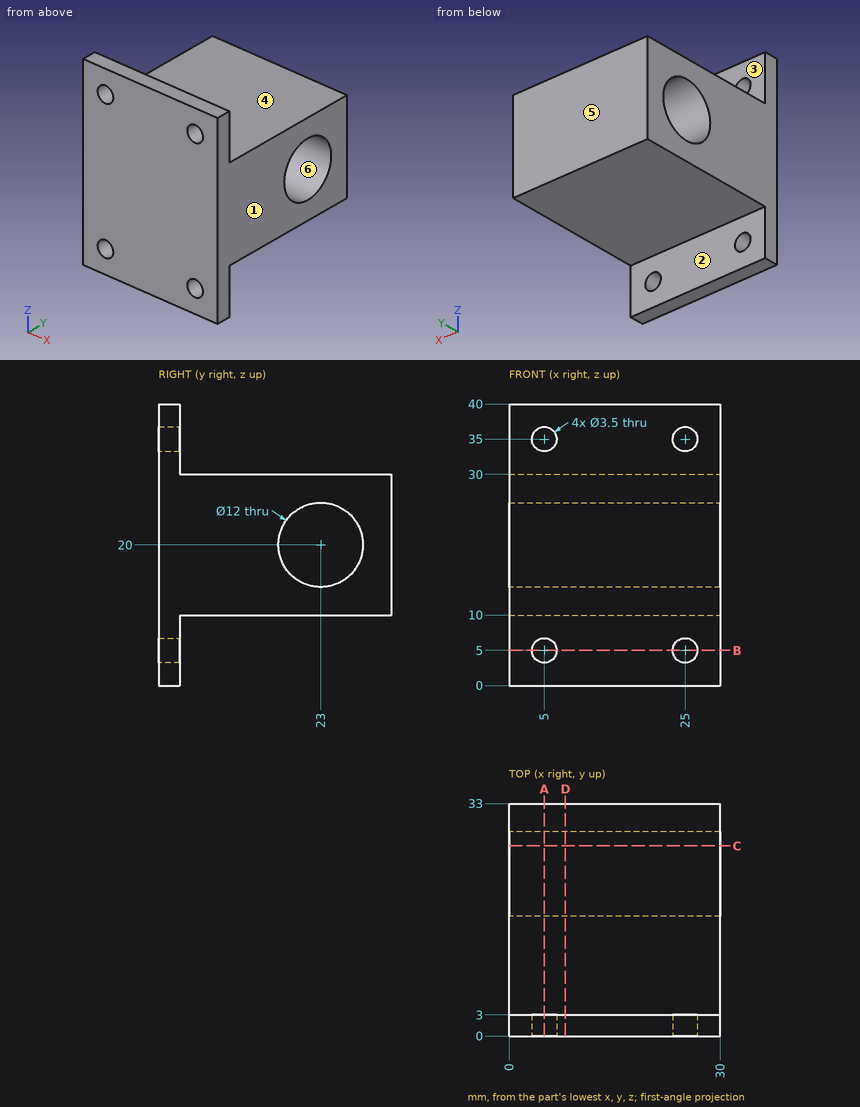
Check sheet for the drawn part. Datum: minimum x, y, z corner. Units: mm. A direction names the side the tool comes from. Coordinates: 2 decimals unless noted, no trailing zeros. Write each loop counter-clockwise with the first axis right and the second up, starting at its lowest first coordinate (ties: lowest second). Pieces come first, ordered by that corner, then holes. Notation, with made-up numbers: (-10, 85) - (46, 85) arc R21 ccw to (46, 100) - close; hole circle Ø7 at (26.25, 47.5). An arc over 180 degrees is marked (long way). Answer as a JSON object with one key per item and string values.
(1) Gauge pin test, flat ends, axial feed: pin 1 Ø4.5 at (x, z) = (5, 5) entering from +Y; pin 2 Ø12 at (x, y) = (4, 17) entering from -Z; pin 3 Ø15 at (x, y) = (18.5, 23.5) entering from +Z. Record the tip position at first contact, or that the pin passes through.
Report:
{"pin 1": "y = 3", "pin 2": "z = 10", "pin 3": "z = 30"}
(2) Cross-section at C-C on y = 27. Record the cut outline in (x, z).
Report:
{"outline": "(0, 10) - (30, 10) - (30, 15.53) - (0, 15.53) - close; (0, 24.47) - (30, 24.47) - (30, 30) - (0, 30) - close"}
(3) Mould release check, pull along Z, two halves, no side actions. Record for the marked faces 4, 5 and 6: pulls with the +Z half, pulls with the -Z half, needs draft (parallel to the pull), parting line crosses it, or undercut.
Report:
{"face 4": "pulls with the +Z half", "face 5": "needs draft", "face 6": "undercut"}
(4) Cross-section at D-D on x = 8. Record the cut outline in (y, z), plus the area to 3 significant figures.
Report:
{"outline": "(0, 0) - (3, 0) - (3, 10) - (33, 10) - (33, 30) - (3, 30) - (3, 40) - (0, 40) - close; hole circle Ø12 at (23, 20)", "area": "607 mm^2"}
(5) Cross-section at B-B on z = 5. Record the cut outline in (x, y).
Report:
{"outline": "(0, 0) - (3.25, 0) - (3.25, 3) - (0, 3) - close; (6.75, 0) - (23.25, 0) - (23.25, 3) - (6.75, 3) - close; (26.75, 0) - (30, 0) - (30, 3) - (26.75, 3) - close"}
(6) Cross-section at A-A on x = 5. Record the cut outline in (y, z), plus the area to 3 significant figures.
Report:
{"outline": "(0, 0) - (3, 0) - (3, 3.25) - (0, 3.25) - close; (0, 6.75) - (3, 6.75) - (3, 10) - (33, 10) - (33, 30) - (3, 30) - (3, 33.25) - (0, 33.25) - close; (0, 36.75) - (3, 36.75) - (3, 40) - (0, 40) - close; hole circle Ø12 at (23, 20)", "area": "586 mm^2"}
(7) Tool access check on the marked faces 1, 2 and 3. Record the directions out of +Z, -Z, +X, -X, +Y, -Y that give a thin tool (end or side, any length) a straight path to the whole face; none if there is none.
Report:
{"face 1": "+Z, -Z, +X, +Y, -Y", "face 2": "-Z, +X, -X, +Y", "face 3": "+Z, +X, -X, +Y"}
(8) Thickness scan on line 1 along X through (y, z) = (1.25, 35); line 2 along Y through (x, z) = (15.25, 20); line 3 along Y through (x, z) = (3.5, 37). Record the ranges inside material, lowest first.
Report:
{"line 1": "0 to 3.25, 6.75 to 23.25, 26.75 to 30", "line 2": "0 to 17, 29 to 33", "line 3": "0 to 3"}
